Input: part model. Units: mm. Frame: model coordinates. A direction names the side the tool comes from. Coordinates: 2 decimals unless noted, no trailing zeros. Order: outer loops, then holes, each group sorted by start corner. A loop starts at its lowest first (then second) coordinate and runs counter-clockwise, first axis right, second up. Notation, with made-up numbers: (88, 0) -> (96, 0) arc R9 ccw to (96, 16) -> close; hole circle Ø4 at (-23.75, 10). An arc over 180 degrees is marked (long way). Write each question's results on one line, items separated by ' | '.
```python
from build123d import *

# Parameters (mm, degrees)
F0_W     = 71.338967
F0_H     = 42.17276
F1_DEPTH = 3.048
F2_W     = 71.338967
F2_H     = 42.17276
F2_W_2   = 66.609312
F2_H_2   = 37.443103
F3_DEPTH = 6.604
F4_W     = 22.226787
F4_H     = 15.836691
F4_W_2   = 19.411293
F4_H_2   = 12.809481
F5_DEPTH = 13.97


with BuildPart() as f1:
    # F0 (on Front) → F1 (new body)
    with BuildSketch(Plane.XZ):
        with Locations((-3.153104, 3.547242)):
            Rectangle(F0_W, F0_H)
    extrude(amount=F1_DEPTH)

    # F2 (on face) → F3 (join)
    with BuildSketch(Plane.XZ.offset(3.048)):
        with Locations((-3.153104, 3.547242)):
            Rectangle(F2_W, F2_H)
        with Locations((-3.547242, 3.941378)):
            Rectangle(F2_W_2, F2_H_2, mode=Mode.SUBTRACT)
    extrude(amount=F3_DEPTH)

    # F4 (on face) → F5 (join)
    with BuildSketch(Plane.XZ.offset(3.048)):
        with Locations((-3.042677, 2.090226)):
            Rectangle(F4_W, F4_H)
        with Locations((-3.005302, 1.970689)):
            Rectangle(F4_W_2, F4_H_2, mode=Mode.SUBTRACT)
    extrude(amount=F5_DEPTH)


solid = f1.part
```
(1) Cut plane C-C, the plane x = -15.5. Return loops of the section in (y, z), plus the area to 3 significant figures.
Return value:
outline: (-9.65, -17.54) -> (0, -17.54) -> (0, 24.63) -> (-9.65, 24.63) -> (-9.65, 22.66) -> (-3.05, 22.66) -> (-3.05, -14.78) -> (-9.65, -14.78) -> close | area: 160 mm2
(2) Pin query (flat end, axial travel): P1, Ø6, axis at x = -8, z = -9, coming from the +Y side; P2, Ø12, axis at x = -26.5, z = 4, coming from the -Y side; P3, Ø1.5, axis at x = -2.5, y = -11, coming from the +Z side. Return the tip coordinate at first contact, or that it passes through.
Return value:
P1: y = 0 | P2: y = -3.05 | P3: z = 10.01
(3) Cut plane A-A, the plane y = -7.75. Return loops of the section in (x, z), plus the area to 3 significant figures.
Return value:
outline: (-38.82, -17.54) -> (32.52, -17.54) -> (32.52, 24.63) -> (-38.82, 24.63) -> close; (-14.16, -5.83) -> (8.07, -5.83) -> (8.07, 10.01) -> (-14.16, 10.01) -> close; hole (-36.85, -14.78) -> (29.76, -14.78) -> (29.76, 22.66) -> (-36.85, 22.66) -> close; hole (-12.71, -4.43) -> (6.7, -4.43) -> (6.7, 8.38) -> (-12.71, 8.38) -> close | area: 618 mm2
(4) Line query: line 1 along Z through (x, y) = (-11.5, -8.5); line 2 along X through (y, z) = (-4.5, -0.5); line 3 along X through (y, z) = (-15.5, -1.5). Output: solid intervals per line, ascending. Write a range as from..to.
Return value:
line 1: -17.54..-14.78, -5.83..-4.43, 8.38..10.01, 22.66..24.63 | line 2: -38.82..-36.85, -14.16..-12.71, 6.7..8.07, 29.76..32.52 | line 3: -14.16..-12.71, 6.7..8.07
(5) Cut plane B-B, the plane y = -14.25. Return loops of the section in (x, z).
Return value:
outline: (-14.16, -5.83) -> (8.07, -5.83) -> (8.07, 10.01) -> (-14.16, 10.01) -> close; hole (-12.71, -4.43) -> (6.7, -4.43) -> (6.7, 8.38) -> (-12.71, 8.38) -> close
(6) Mould query, pull axis Z, two halves, no side actions, for faces 3 (the face through (-3, -9.652, -15)), 4 (the face through (-4, -5, -17.539)), 5 (the face through (-4, -5, 24.634)), 6 (the face through (-3, -3.048, 2)). Classes: +Z half, -Z half, draft (parallel to the pull), parting line (faces both ways), or undercut.
Return value:
face 3: draft | face 4: -Z half | face 5: +Z half | face 6: undercut
(7) Reachability of faces 1 (the face through (32.516, -5, 3)), 2 (the face through (8.071, -10, 2)) from +Z, -Z, +X, -X, +Y, -Y: full face, straight path, thin tool, end or side. Return the list, or none.
Return value:
face 1: +Z, -Z, +X, +Y, -Y | face 2: -Y
(8) Cut plane D-D, the plane z = 15.5. Return loops of the section in (x, y).
Return value:
outline: (-38.82, -9.65) -> (-36.85, -9.65) -> (-36.85, -3.05) -> (29.76, -3.05) -> (29.76, -9.65) -> (32.52, -9.65) -> (32.52, 0) -> (-38.82, 0) -> close
